Read the model definition and answer for the solid it produces. Units are mm, in the model's axes. A direction names the side the tool comes from. Coordinates: 2 decimals unless noted, no trailing zeros. Loops run counter-clockwise (first coordinate to the right, second up) from the corner with the lowest first, then second, coordinate; pieces in that order, holes last. Notation, with made-up numbers: (12.25, 9.5) - (27.25, 9.5) arc R18 cw to (27.25, 30.5) - close; hole circle Ø7 at (30.25, -30). An arc over 180 degrees is marked (long way). One line per question, with ' | ' between items. Start each with the question number.
```python
from build123d import *

# Parameters (mm, degrees)
BOSS_EXTRUDE1_DEPTH = 2.794
FILLET1_R           = 2.54


with BuildPart() as part:
    # Sketch1 → Boss-Extrude1 (new body)
    with BuildSketch(Plane.XY):
        Polygon((-4.201711417, 0), (75.173288583, 0), (77.967288583, 0), (77.967288583, 6.35), (75.173288583, 6.35), (75.173288583, 15.875), (60.885788583, 15.875), (60.885788583, 6.35), (10.085788583, 6.35), (10.085788583, 15.875), (-4.201711417, 15.875), (-4.201711417, 6.35), (-6.995711417, 6.35), (-6.995711417, 0.062112437), align=None)
    extrude(amount=BOSS_EXTRUDE1_DEPTH)

    # Fillet1
    fillet1_edges = [part.edges().sort_by_distance(p)[0] for p in [
        (-4.201711417, 15.875, 1.397),
        (75.173288583, 15.875, 1.397),
    ]]
    fillet(fillet1_edges, radius=FILLET1_R)


solid = part.part
```
1) Find the intervals of material crossed by line 1 along X through (y, z) = (10, 2.1); line 2 along Y through (x, z) = (24, 0.45); line 3 along X through (y, z) = (15, 1.3), in increasing order. Write a range as from..to.
2) The part is cut by section C-C on x = 11. Write down the section's boundary in (y, z), and give its area (3 significant figures).
3) The part is cut by section B-B on z = 1. Write down the section's boundary in (x, y) (3 decimals).
4) Which of the six approach directions +Z, -Z, +X, -X, +Y, -Y give full straight-line access (tool end or side, diameter ignored) to faces 4 (the cylindrical face through (74.45, 15.11, 1.42)), 5 (the flat face through (60.886, 11, 1)), 6 (the flat face through (-4.202, 10, 1))?
5) The part is cut by section A-A on y = 8. Write down the section's boundary in (x, z), and give its area (3 significant figures).
6) The mould has two halves that part along X. Classify faces 1 (the flat face through (77, 6.35, 1)), 2 (the flat face through (75.173, 10, 1)), 3 (the flat face through (10.086, 11, 1)): released by +X, released by -X, zero draft, split by the parting line, or undercut.
7) Given pin 1 Ø1.4 at (x, z) = (76.5, 1) entering from +Y; pin 2 Ø1.5 at (y, z) = (13.5, 2) entering from +X; pin 3 Ø2 at (x, y) = (18.5, 7.5) entering from -Z, each flat-ended and moving along its own axis, determine where each tip first touches the part or whether it passes through.
Answer below:
1) line 1: -4.2..10.09, 60.89..75.17 | line 2: 0..6.35 | line 3: -3.58..10.09, 60.89..74.55
2) outline: (0, 0) - (6.35, 0) - (6.35, 2.79) - (0, 2.79) - close | area: 17.7 mm2
3) outline: (-6.996, 0.062) - (-4.202, 0) - (77.967, 0) - (77.967, 6.35) - (75.173, 6.35) - (75.173, 13.335) arc R2.54 ccw to (72.633, 15.875) - (60.886, 15.875) - (60.886, 6.35) - (10.086, 6.35) - (10.086, 15.875) - (-1.662, 15.875) arc R2.54 ccw to (-4.202, 13.335) - (-4.202, 6.35) - (-6.996, 6.35) - close
4) face 4: +Z, -Z, +X, +Y | face 5: +Z, -Z, +Y | face 6: +Z, -Z, -X, +Y
5) outline: (-4.2, 0) - (10.09, 0) - (10.09, 2.79) - (-4.2, 2.79) - close; (60.89, 0) - (75.17, 0) - (75.17, 2.79) - (60.89, 2.79) - close | area: 79.8 mm2
6) face 1: zero draft | face 2: released by +X | face 3: undercut
7) pin 1: y = 6.35 | pin 2: x = 75.17 | pin 3: through
